```python
from build123d import *

# Parameters (mm, degrees)
SKETCH1_W           = 254
SKETCH1_H           = 6.35
BOSS_EXTRUDE1_DEPTH = 304.8
CUT_EXTRUDE1_DEPTH  = 304.8
CUT_EXTRUDE2_DEPTH  = 397.811494919
CUT_EXTRUDE3_REACH  = 398.811
FILLET2_R           = 2.54


with BuildPart() as part:
    # Sketch1 → Boss-Extrude1 (new body)
    with BuildSketch(Plane.XY):
        with Locations((-127, 3.175)):
            Rectangle(SKETCH1_W, SKETCH1_H)
    extrude(amount=BOSS_EXTRUDE1_DEPTH)

    # Sketch2 → Cut-Extrude1 (cut)
    with BuildSketch(Plane(origin=(0, 6.35, 0), x_dir=(1, 0, 0), z_dir=(0, 1, 0))):
        Polygon((-177.8, -304.8), (-254, 0), (-254, -304.8), align=None)
    extrude(amount=-CUT_EXTRUDE1_DEPTH, mode=Mode.SUBTRACT)

    # Sketch4 → Cut-Extrude2 (cut, through all)
    with BuildSketch(Plane(origin=(0, 6.35, 0), x_dir=(1, 0, 0), z_dir=(0, 1, 0))):
        Polygon((-76.2, -127), (-76.2, 0), (0, 0), (0, -304.8), (-76.2, -304.8), (-76.2, -177.8), align=None)
    extrude(amount=-CUT_EXTRUDE2_DEPTH, mode=Mode.SUBTRACT)

    # Sketch7 → Cut-Extrude3 (cut, up to next)
    with BuildSketch(Plane(origin=(0, 0, 0), x_dir=(-1, 0, 0), z_dir=(0, -1, 0)), mode=Mode.PRIVATE) as cut_extrude3_sk1:
        with BuildLine():
            ThreePointArc((98.637189175, -117.047779868), (92.943689479, -119.991917487), (88.9, -115.0187434))
            Line((88.9, -115.0187434), (88.9, -30.48))
            ThreePointArc((88.9, -30.48), (90.387897552, -26.887897552), (93.98, -25.4))
            Line((93.98, -25.4), (130.811699734, -25.4))
            ThreePointArc((130.811699734, -25.4), (135.061047052, -27.696217075), (135.468888909, -32.509036468))
            Line((135.468888909, -32.509036468), (98.637189175, -117.047779868))
        make_face()
    cut_extrude3_tool1 = extrude(cut_extrude3_sk1.sketch, amount=-CUT_EXTRUDE3_REACH, mode=Mode.PRIVATE) & part.part
    # Sketch7 → Cut-Extrude3 (cut, up to next)
    with BuildSketch(Plane(origin=(0, 0, 0), x_dir=(-1, 0, 0), z_dir=(0, -1, 0)), mode=Mode.PRIVATE) as cut_extrude3_sk2:
        with BuildLine():
            Line((198.646676859, -131.504754308), (155.51638644, -32.509036468))
            ThreePointArc((155.51638644, -32.509036468), (155.924228297, -27.696217075), (160.173575615, -25.4))
            Line((160.173575615, -25.4), (228.052795494, -25.4))
            ThreePointArc((228.052795494, -25.4), (232.056879119, -27.353705976), (232.981119395, -31.712080975))
            Line((232.981119395, -31.712080975), (208.232189935, -130.707798815))
            ThreePointArc((208.232189935, -130.707798815), (203.724773416, -134.538250504), (198.646676859, -131.504754308))
        make_face()
    cut_extrude3_tool2 = extrude(cut_extrude3_sk2.sketch, amount=-CUT_EXTRUDE3_REACH, mode=Mode.PRIVATE) & part.part
    # Sketch7 → Cut-Extrude3 (cut, up to next)
    with BuildSketch(Plane(origin=(0, 0, 0), x_dir=(-1, 0, 0), z_dir=(0, -1, 0)), mode=Mode.PRIVATE) as cut_extrude3_sk3:
        with BuildLine():
            ThreePointArc((156.152382169, -284.48), (156.152382169, -289.56), (151.752973118, -292.1))
            Line((151.752973118, -292.1), (93.98, -292.1))
            ThreePointArc((93.98, -292.1), (90.387897552, -290.612102448), (88.9, -287.02))
            Line((88.9, -287.02), (88.9, -186.954275256))
            ThreePointArc((88.9, -186.954275256), (92.665199251, -182.047372059), (98.379409051, -184.414275256))
            Line((98.379409051, -184.414275256), (156.152382169, -284.48))
        make_face()
    cut_extrude3_tool3 = extrude(cut_extrude3_sk3.sketch, amount=-CUT_EXTRUDE3_REACH, mode=Mode.PRIVATE) & part.part
    # Sketch7 → Cut-Extrude3 (cut, up to next)
    with BuildSketch(Plane(origin=(0, 0, 0), x_dir=(-1, 0, 0), z_dir=(0, -1, 0)), mode=Mode.PRIVATE) as cut_extrude3_sk4:
        with BuildLine():
            Line((173.146484204, -271.050621738), (198.919755106, -167.957538129))
            ThreePointArc((198.919755106, -167.957538129), (197.995514831, -163.59916313), (193.991431206, -161.645457154))
            Line((193.991431206, -161.645457154), (108.69734073, -161.645457154))
            ThreePointArc((108.69734073, -161.645457154), (104.297931679, -164.185457154), (104.297931679, -169.265457154))
            Line((104.297931679, -169.265457154), (163.818751252, -272.358540762))
            ThreePointArc((163.818751252, -272.358540762), (168.923568535, -274.849325912), (173.146484204, -271.050621738))
        make_face()
    cut_extrude3_tool4 = extrude(cut_extrude3_sk4.sketch, amount=-CUT_EXTRUDE3_REACH, mode=Mode.PRIVATE) & part.part
    # Sketch7 → Cut-Extrude3 (cut, up to next)
    with BuildSketch(Plane(origin=(0, 0, 0), x_dir=(-1, 0, 0), z_dir=(0, -1, 0)), mode=Mode.PRIVATE) as cut_extrude3_sk5:
        with BuildLine():
            ThreePointArc((106.347495425, -148.945457154), (102.098148107, -146.649240078), (101.69030625, -141.836420686))
            Line((101.69030625, -141.836420686), (140.835448499, -51.987699072))
            ThreePointArc((140.835448499, -51.987699072), (145.492637674, -48.93673554), (150.14982685, -51.987699072))
            Line((150.14982685, -51.987699072), (189.2949691, -141.836420686))
            ThreePointArc((189.2949691, -141.836420686), (188.887127243, -146.649240078), (184.637779925, -148.945457154))
            Line((184.637779925, -148.945457154), (106.347495425, -148.945457154))
        make_face()
    cut_extrude3_tool5 = extrude(cut_extrude3_sk5.sketch, amount=-CUT_EXTRUDE3_REACH, mode=Mode.PRIVATE) & part.part
    add(cut_extrude3_tool1.solids().sort_by_distance((-105.779096, 0, 61.624334))[0], mode=Mode.SUBTRACT)
    add(cut_extrude3_tool2.solids().sort_by_distance((-197.184891, 0, 64.864333))[0], mode=Mode.SUBTRACT)
    add(cut_extrude3_tool3.solids().sort_by_distance((-112.936879, 0, 251.56545))[0], mode=Mode.SUBTRACT)
    add(cut_extrude3_tool4.solids().sort_by_distance((-156.854236, 0, 201.939756))[0], mode=Mode.SUBTRACT)
    add(cut_extrude3_tool5.solids().sort_by_distance((-145.492638, 0, 113.262605))[0], mode=Mode.SUBTRACT)

    # Fillet2
    fillet2_edges = [part.edges().sort_by_distance(p)[0] for p in [
        (-215.9, 0, 152.4),
        (-215.9, 6.35, 152.4),
        (-177.8, 3.175, 304.8),
        (-165.1, 0, 0),
        (-165.1, 6.35, 0),
        (-127, 6.35, 304.8),
        (-127, 0, 304.8),
        (-76.2, 6.35, 152.4),
        (-76.2, 3.175, 304.8),
        (-76.2, 3.175, 0),
        (-76.2, 0, 152.4),
        (-254, 3.175, 0),
    ]]
    fillet(fillet2_edges, radius=FILLET2_R)


solid = part.part
```
Design review of the part built by this model. Coordinates are the model's own, in mm. Coordinates: 2 decimals unless noted, no trailing zeros. Answer as a JSON object with one key per item and string values.
Q1. The part is to be moulded in two halves that separate along X. For faces 1 (the flat face through (-152, 3, 161.645)), 2 (the flat face through (-152, 6.35, 152)), 3 (the cylindrical face through (-215.568, 0.764, 150.742)), say which applies: +X half, -X half, draft (parallel to the pull), parting line (faces both ways), or undercut.
Answer block:
{"face 1": "undercut", "face 2": "draft", "face 3": "-X half"}
Q2. Clearance check with a flat-ended pin moving along its axis: pin 1 Ø3 at (y, z) = (5.5, 210) entering from +X. State where the tip first meets the part, or that it passes through.
Answer block:
{"pin 1": "stops at x = -76.21"}
Q3. To check wall thickness, follow L1, parallel to X at y = 2.25, z = 105; L2, parallel to X at y = 3, z = 188; L3, parallel to Z at x = -113.5, y = 2.75. State the ranges of each line that lie inside material, in increasing order.
Answer block:
{"L1": "x = -227.73 to -214.66, -187.1 to -173.25, -117.74 to -103.89, -88.9 to -76.22", "L2": "x = -207 to -193.91, -115.11 to -100.45, -88.9 to -76.2", "L3": "z = 0 to 25.4, 82.93 to 114.73, 148.95 to 161.65, 185.2 to 210.6, 292.1 to 304.8"}
Q4. Take a section at A-A on y = 5. Give the number of separate pieces and of enclosed holes in the cut face, plus the area to 3 significant figures.
Answer block:
{"separate pieces": "1", "enclosed holes": "5", "area": "19,300 mm^2"}
